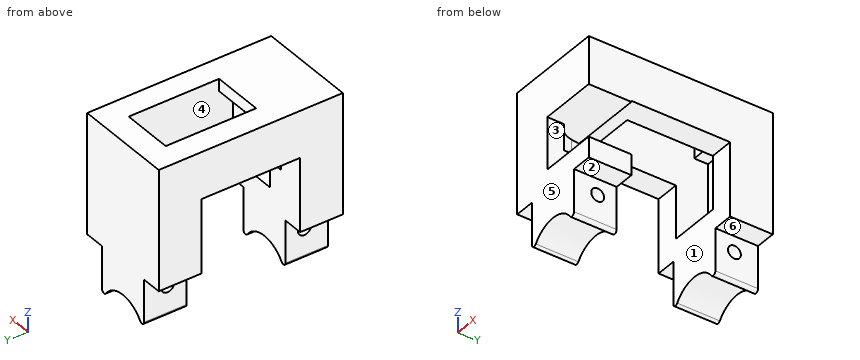
Autodesk Inventor part; units mm, degrees
ref_plane "Work Plane3" through (-12.7635, -20.2311, -42.672) normal (0, -1, 0) x (1, 0, 0)
ref_plane "Work Plane4" through (-6.2203, -16.256, -6.731) normal (0, 0, -1) x (0, 1, 0)
ref_plane "YZ Plane" through (0, 0, 0) normal (1, 0, 0) x (0, 1, 0)
sketch "Servo Containment" plane through (0, 0, 0) normal (0, 0, 1) x (1, 0, 0)
  line L0 (-22.2827, 48.831) -> (-35.4907, 48.831)
  line L1 (-35.4907, 48.831) -> (-35.4907, 18.351)
  line L2 (-35.4907, 18.351) -> (-22.2827, 18.351)
  line L3 (-22.2827, 18.351) -> (-22.2827, 48.831)
  line L4 (-22.2827, 45.275) -> (-35.4907, 45.275)
  line L5 (-35.4907, 45.275) -> (-35.4907, 21.907)
  line L6 (-35.4907, 21.907) -> (-22.2827, 21.907)
  line L7 (-22.2827, 21.907) -> (-22.2827, 45.275)
  line L8 (-28.8867, 18.351) -> (-28.8867, 21.907) construction
  line L9 (-28.8867, 45.275) -> (-28.8867, 48.831) construction
  line L10 (-28.8867, 21.907) -> (-28.8867, 27.749)
  point P0 (-28.8867, 33.0211)
  dimension "d0" = 13.208
  dimension "d1" = 30.48
  dimension "d2" = 23.368
  dimension "d4" = 5.842
sketch "zdstj" plane through (0, 0, 0) normal (0, 0, 1) x (1, 0, 0)
  line L0 (-10.4838, -7.9303) -> (-9.9261, -12.0195)
  arc A0 (-9.9261, -12.0195) -> (1.399, -12.0195) centre (-4.2636, -11.2472) ccw
  point P0 (-6.5265, -10.9007)
ref_plane "Work Plane1" through (0, 0, 0) normal (0, 0, 1) x (1, 0, 0)
sketch "Sketch1" plane through (0, 0, 0) normal (0, 0, 1) x (1, 0, 0)
  arc A0 (6.2203, -7.2241) -> (-6.2203, -7.2241) centre (0, 3.556) ccw
  line L0 (2.032, 8.0666) -> (2.032, -8.723)
  arc A1 (4.826, -6.5243) -> (4.826, 13.6363) centre (0, 3.556) ccw
  arc A2 (2.032, -8.723) -> (-2.032, -8.723) centre (0, 3.556) ccw
  line L1 (-12.7635, 27.3431) -> (12.7635, 27.3431)
  line L2 (12.7635, 27.3431) -> (12.7635, -20.2311)
  line L3 (12.7635, -20.2311) -> (-12.7635, -20.2311)
  line L4 (-12.7635, -20.2311) -> (-12.7635, 27.3431)
  arc A3 (-5.6626, -11.3133) -> (5.6626, -11.3133) centre (0, -10.541) ccw
  line L5 (-6.2203, -7.2241) -> (-5.6626, -11.3133)
  line L6 (-6.2203, -7.2241) -> (-6.2203, -20.2311)
  circle A4 centre (0, 3.556) radius 12.7635
  line L7 (14.097, 3.556) -> (0, 3.556)
  line L8 (6.604, 24.638) -> (-6.604, 24.638)
  line L9 (-6.604, 24.638) -> (-6.604, -5.842)
  line L10 (-6.604, -5.842) -> (6.604, -5.842)
  line L11 (6.604, -5.842) -> (6.604, 24.638)
  line L12 (6.604, 21.082) -> (-6.604, 21.082)
  line L13 (-6.604, 21.082) -> (-6.604, -2.286)
  line L14 (-6.604, -2.286) -> (6.604, -2.286)
  line L15 (6.604, -2.286) -> (6.604, 21.082)
  line L16 (0, -5.842) -> (0, -2.286) construction
  line L17 (0, 21.082) -> (0, 24.638) construction
  line L18 (0, -2.286) -> (0, 3.556)
  line L19 (10.7801, 9.7763) -> (14.8693, 9.2186)
  arc A5 (14.8693, 9.2186) -> (14.8693, -2.1066) centre (14.097, 3.556) cw
  point P0 (0, 0)
  point P1 (0, 3.556)
  point P2 (0, -19.05)
  point P3 (12.7635, 27.3431)
  point P4 (-12.7635, -20.2311)
  point P5 (6.604, 14.4782)
  point P6 (11.1751, 9.7224)
  point P7 (12.7635, 9.5058)
  point P8 (-12.7635, 3.556)
  point P9 (-6.604, 14.4782)
  point P10 (-6.604, 14.1054)
  point P11 (6.604, 14.1054)
  point P12 (-6.2203, -7.5892)
ref_plane "Work Plane2" through (-12.7635, 27.3431, -23.876) normal (0, 1, 0) x (1, 0, 0)
sketch "Sketch2" plane through (-12.7635, 27.3431, -23.876) normal (0, 1, 0) x (1, 0, 0)
  arc A0 (17.5895, 10.6426) -> (7.9375, 10.6426) centre (12.7635, 10.6426) ccw
  line L0 (17.5895, 0) -> (17.5895, 10.6426)
  line L1 (7.9375, 10.6426) -> (7.9375, 0)
  arc A1 (20.2819, 10.6426) -> (5.2451, 10.6426) centre (12.7635, 10.6426) ccw
  line L2 (20.2819, 10.6426) -> (20.2819, 0)
  line L3 (20.2819, 10.6426) -> (20.2819, 0)
  line L4 (25.527, -5.08) -> (25.527, 18.796)
  line L5 (0, 18.796) -> (25.527, 18.796)
  line L6 (0, -5.08) -> (0, 18.796)
  line L7 (5.2451, 0) -> (5.2451, 10.6426)
  arc A2 (20.2819, 10.6426) -> (5.2451, 10.6426) centre (12.7635, 10.6426) ccw
  circle A3 centre (12.7635, 10.6426) radius 7.5184
  line L8 (20.2819, 0) -> (20.32, 0)
  line L9 (20.32, 0) -> (20.32, -5.08)
  line L10 (25.527, -5.08) -> (20.32, -5.08)
  line L11 (5.207, -5.08) -> (0, -5.08)
  line L12 (5.207, 0) -> (5.207, -5.08)
  line L13 (5.207, 0) -> (5.2451, 0)
  line L14 (5.207, -5.08) -> (20.32, -5.08)
  line L15 (20.2819, 0) -> (20.2819, -5.08)
  line L16 (5.2451, 0) -> (5.2451, -5.08)
  point P0 (12.7635, -23.876)
  point P1 (20.2819, 10.6426)
  point P2 (5.2451, 10.6426)
ref_plane "Work Plane3" through (-12.7635, -20.2311, -42.672) normal (0, -1, 0) x (1, 0, 0)
extrude "Extrusion1" add sketch "Sketch2" against normal up to surface (47.5742 mm away) contours A3 L2 L15 L14 L16 L7
fillet "Fillet1" radius 0.762 2 edges at (-7.5184, 3.556, -34.5186) (7.5184, 3.556, -34.5186)
extrude "Extrusion2" add sketch "Sketch1" against normal up to surface (18.796 mm away) contours A4 L11 L8 L9 L4 L1 L2 L19 | A4 L9 L12 L11 | L3 L4 A4 L6 | L12 L9 L8 L11
sketch "Sketch3" plane through (-7.5184, -20.2311, -23.876) normal (-1, 0, 0) x (0, 0, 1)
  circle A0 centre (0.9779, 6.1087) radius 1.6637
  circle A1 centre (0.9779, 41.4655) radius 1.6637
  point P0 (23.876, 20.2311)
extrude "Extrusion3" cut sketch "Sketch3" against normal blind 25.4
sketch "Sketch7" plane through (0, 3.556, -18.796) normal (0, 0, 1) x (1, 0, 0)
  circle A0 centre (0, 0) radius 12.7635
  line L0 (12.7635, 23.7871) -> (12.7635, -23.7871)
  line L1 (12.7635, -23.7871) -> (-12.7635, -23.7871)
  line L2 (-12.7635, 23.7871) -> (12.7635, 23.7871)
  line L3 (-12.7635, -23.7871) -> (-12.7635, 23.7871)
  line L4 (-6.2203, -11.1452) -> (-6.2203, -23.7871)
  arc A1 (-5.6626, -14.8693) -> (5.6626, -14.8693) centre (0, -14.097) ccw
  line L5 (-6.2203, -10.7801) -> (-5.6626, -14.8693)
  line L6 (-2.032, -23.7871) -> (-2.032, 22.087)
  line L7 (0, -23.7871) -> (0, 23.7871)
  line L8 (12.7635, 5.9498) -> (11.1751, 6.1664)
  point P0 (0, -3.556)
  point P1 (-2.032, -19.4386)
  point P2 (-6.1664, -11.1751)
  point P3 (12.7635, 0)
  point P4 (-2.032, -12.6007)
  dimension "d17" = 2.032
extrude "Extrusion4" add sketch "Sketch7" along normal blind 5.334 contours L0 L1 L7 A0 | A0 L8 L0 | L7 A1 L6 A0 | L6 A1 L5 A0 | L7 L1 L6 A1 | L5 A1 L6 L1 L4 A0
extrude "Extrusion5" add sketch "Sketch7" along normal up to surface (18.796 mm away) contours L5 A1 L6 L1 L4 A0
extrude "Extrusion6" cut sketch "Sketch7" along normal mid plane 55.5625 contours A0 L7 | A0 L6 L7 | A0 L6
ref_plane "Work Plane4" through (-6.2203, -16.256, -6.731) normal (0, 0, -1) x (0, 1, 0)
extrude "Extrusion7" add sketch "Sketch7" along normal up to surface (12.065 mm away) contours L6 A1 L5 A0
ref_plane "Work Plane5" through (0, 0, 9.144) normal (0, 0, 1) x (1, 0, 0)
sketch "Sketch14" plane through (0, 0, 9.144) normal (0, 0, 1) x (1, 0, 0)
  line L0 (-12.7635, -20.2311) -> (-12.7635, 27.3431)
  line L1 (12.7635, 27.3431) -> (-12.7635, 27.3431)
  line L2 (12.7635, 27.3431) -> (12.7635, -20.2311)
  line L3 (12.7635, -20.2311) -> (-12.7635, -20.2311)
  line L4 (-6.604, 24.638) -> (-6.604, -5.842)
  line L5 (-6.604, -5.842) -> (6.604, -5.842)
  line L6 (6.604, -5.842) -> (6.604, 24.638)
  line L7 (6.604, 24.638) -> (-6.604, 24.638)
  line L8 (6.604, 21.082) -> (-6.604, 21.082)
  line L9 (-6.604, -2.286) -> (6.604, -2.286)
  arc A0 (11.1751, 9.7224) -> (-12.7635, 3.556) centre (0, 3.556) ccw
  line L10 (0, 16.3195) -> (12.7635, 16.3195)
  arc A1 (-2.032, -9.0447) -> (12.7635, 3.556) centre (0, 3.556) ccw
  line L11 (0, -9.2075) -> (12.7635, -9.2075)
  point P0 (0, 0)
extrude "Extrusion8" add sketch "Sketch14" against normal up to surface (9.144 mm away) contours L0 A0 L4 L5 L6 L10 L2 A1 L11 L3 | L0 L1 L2 L10 L6 L7 L4 A0 | L11 A1 L2
extrude "Extrusion9" add sketch "Sketch14" along normal blind 3.175 contours L0 A0 L4 L5 L6 L10 L2 A1 L11 L3 | L0 L1 L2 L10 L6 L7 L4 A0 | L11 A1 L2 | L4 L7 L6 L8 | L9 L6 L5 L4
extrude "Extrusion10" cut sketch "Sketch14" against normal up to surface (22.606 mm away) contours A0 L6 L9 L4 | L4 L8 L6 L10 A0 | L4 L7 L6 L8 | L10 L6 A0
sketch "Sketch15" plane through (0, 3.556, -18.796) normal (0, 0, -1) x (-1, 0, 0)
  line L0 (0, -12.7635) -> (-22.033, -12.7635)
  line L1 (-22.033, -12.7635) -> (-22.033, 12.7635)
  line L2 (0, 12.7635) -> (-22.033, 12.7635)
  line L3 (-22.033, -12.7635) -> (27.2623, -12.7635)
  line L4 (27.2623, -12.7635) -> (27.2623, 12.7635)
  line L5 (27.2623, 12.7635) -> (-22.033, 12.7635)
  line L6 (-22.033, 12.7635) -> (-22.033, -12.7635)
  point P0 (0, -3.556)
  point P1 (0, -12.7635)
extrude "Extrusion11" cut sketch "Sketch15" along normal blind 14.2875 and the other way blind 19.0627
properties part number "Servo Mount V4"
Here's how the part is built. I have some questions about the finished solid (model axes, mm). Face numbers are marked on the shaded views. A direction names the side the tool comes from. Give positions to 0.01 mm unless a question says otherwise; leave off trailing zeros. Write each loop counter-clockwise with the first axis right and the second up, starting at its lowest first coordinate (ties: lowest second). Pieces come first, ordered by that corner, then holes. Notation, with made-up numbers: (63, -15.5) -> (72, -15.5) arc R11 cw to (72, 5.5) -> close; hole circle Ø2 at (-6, 76). An arc over 180 degrees is marked (long way). Use one line per item in the form item = value. Start each with the question number.
1. Imagine slicing it at C-C on z = 3.5. List the corners of the cut face in (x, y) for me.
2. If I drill on L1, parallel to Y at x = -3.5, z = 1; L2, parallel to Y at x = 4.5, z = -24; L3, parallel to Y at x = 4, z = 10.5, over which ranges is the centre line in solid material (lowest first)?
3. On a 3-axis mill with a long thin cutter (end or side, diameter ignored), from which of +Z, -Z, +X, -X, +Y, -Y can I reach the whole of each face in a straight line? I mean the marked faces 1, 2 and 3. Say none if no direction works.
4. Imagine slicing it at B-B on x = 3.75. List the corners of the cut face in (y, z) for me.
5. Imagine slicing it at D-D on y = 4.5. List the corners of the cut face in (x, z) for me.
6. Will these pins go through, and if not, where does the flat tip stop? pin 1 Ø2.5 at (x, y) = (10, 22.5) entering from -Z; pin 2 Ø1.5 at (x, z) = (10, -10.5) entering from -Y; pin 3 Ø8 at (x, y) = (-10, -5) entering from -Z.
7. Thinking about a two-plate mould opening in Y: for the marked faces 4, 5 and 6, which applies, +Y half, -Y half, draft (parallel to the pull), parting line (faces both ways), or undercut?
8. Imagine slicing it at A-A on z = -9. List the corners of the cut face in (x, y) for me, plus the area to 3 significant figures.
Entries:
q1.outline = (-12.76, -20.23) -> (12.76, -20.23) -> (12.76, 27.34) -> (-12.76, 27.34) -> close; hole (-6.6, -5.84) -> (6.6, -5.84) -> (6.6, 24.64) -> (-6.6, 24.64) -> close
q2.L1 = -20.23 to -5.84, 24.64 to 27.34
q2.L2 = -20.23 to -15.37, -12.88 to -9.21, 16.32 to 19.99, 22.48 to 27.34
q2.L3 = -20.23 to -2.29, 21.08 to 27.34
q3.face_1 = -Z, +X, -X
q3.face_2 = -Z, +X, +Y, -Y
q3.face_3 = +X, -Y
q4.outline = (-20.23, -28) -> (-9.21, -28) -> (-9.21, -13.46) -> (-20.23, -13.46) -> close; (-20.23, 0) -> (-9.21, 0) -> (-9.21, 0.27) -> (-5.84, 0.27) -> (-5.84, 9.14) -> (-2.29, 9.14) -> (-2.29, 12.32) -> (-20.23, 12.32) -> close; (16.32, -28) -> (27.34, -28) -> (27.34, 12.32) -> (21.08, 12.32) -> (21.08, 9.14) -> (24.64, 9.14) -> (24.64, -13.46) -> (16.32, -13.46) -> close; hole circle Ø3.33 at (-14.12, -22.9); hole circle Ø3.33 at (21.23, -22.9)
q5.outline = (-12.76, 0.27) -> (-6.6, 0.27) -> (-6.6, 12.32) -> (-12.76, 12.32) -> close; (6.6, 0.27) -> (12.76, 0.27) -> (12.76, 12.32) -> (6.6, 12.32) -> close
q6.pin_1 = -18.8
q6.pin_2 = 16.32
q6.pin_3 = 0.27
q7.face_4 = undercut
q7.face_5 = -Y half
q7.face_6 = draft
q8.outline = (-12.76, -20.23) -> (-2.03, -20.23) -> (-2.03, -9.21) -> (-12.76, -9.21) -> close; (-12.76, 16.32) -> (-6.6, 16.32) -> (-6.6, 24.64) -> (6.6, 24.64) -> (6.6, 16.32) -> (12.76, 16.32) -> (12.76, 27.34) -> (-12.76, 27.34) -> close
q8.area = 290 mm²
